```python
from build123d import *

# Parameters (mm, degrees)
F0_R     = 5.5626
F1_DEPTH = 20.6502
F2_R     = 19.05
F3_DEPTH = 31.75
F5_DEPTH = 68.2762


with BuildPart() as f1:
    # F0 (on Top) → F1 (new body)
    with BuildSketch(Plane.XY):
        with BuildLine():
            ThreePointArc((19.05, 30.048523), (6.35, 30.048523), (0, 19.05))
            Line((0, 19.05), (0, -19.05))
            ThreePointArc((0, -19.05), (6.35, -30.048523), (19.05, -30.048523))
            Line((19.05, -30.048523), (52.045568, -10.998523))
            ThreePointArc((52.045568, -10.998523), (58.395568, 0), (52.045568, 10.998523))
            Line((52.045568, 10.998523), (19.05, 30.048523))
        make_face()
        with Locations((12.7, -19.05)):
            Circle(F0_R, mode=Mode.SUBTRACT)
        with Locations((12.7, 19.05)):
            Circle(F0_R, mode=Mode.SUBTRACT)
        with Locations((45.695568, 0)):
            Circle(F0_R, mode=Mode.SUBTRACT)
    extrude(amount=F1_DEPTH)

    # F2 (on Front) → F3 (join, symmetric)
    with BuildSketch(Plane.XZ):
        with BuildLine():
            Line((12.7, 15.875), (-40.783613, 15.875))
            ThreePointArc((-40.783613, 15.875), (-61.435199, -39.990856), (-9.411603, -10.990385))
            ThreePointArc((-9.411603, -10.990385), (-7.234757, -3.329524), (0, 0))
            Line((0, 0), (12.7, 0))
            Line((12.7, 0), (12.7, 15.875))
        make_face()
        with Locations((-40.783613, -15.875)):
            Circle(F2_R, mode=Mode.SUBTRACT)
    extrude(amount=F3_DEPTH, both=True)

    # F4 (on face) → F5 (cut, through all)
    with BuildSketch(Plane.XY.offset(20.6502)):
        with BuildLine():
            Line((12.7, 13.4874), (12.7, 24.6126))
            ThreePointArc((12.7, 24.6126), (7.1374, 19.05), (12.7, 13.4874))
        make_face()
        with BuildLine():
            ThreePointArc((12.7, -13.4874), (7.1374, -19.05), (12.7, -24.6126))
            Line((12.7, -24.6126), (12.7, -13.4874))
        make_face()
    extrude(amount=-F5_DEPTH, mode=Mode.SUBTRACT)


solid = f1.part
```
Model file for the job. Use its own axes, mm. A direction names the side the tool comes from. Coordinates: 2 decimals unless noted, no trailing zeros. Order: outer loops, then holes, each group sorted by start corner. A loop starts at its lowest first (then second) coordinate and runs counter-clockwise, first axis right, second up. Notation, with made-up numbers: (69, -39) -> (82, -39) arc R16 cw to (82, -27) -> close; hole circle Ø4 at (23.25, 12). An arc over 180 degrees is marked (long way). Return JSON: item names as keys, results as strings.
Item 1: Slice it at C-C (z = -21.5). Write the cut outline in (x, y), then the cut area to 3 significant figures.
Model answer:
{"outline": "(-72.03, -31.75) -> (-58.98, -31.75) -> (-58.98, 31.75) -> (-72.03, 31.75) -> close; (-22.58, -31.75) -> (-9.54, -31.75) -> (-9.54, 31.75) -> (-22.58, 31.75) -> close", "area": "1,660 mm²"}
Item 2: Mould opens along Z. For faces 1 (the face through (-20, 0, 15.875)), 2 (the face through (51, 1.67, 10.18)), 3 (the face through (22, 0, 0)), 4 (the face through (-7.31, -0.44, -3.42)) say: pulls with the +Z half, pulls with the -Z half, needs draft (parallel to the pull), parting line crosses it, or undercut.
Model answer:
{"face 1": "pulls with the +Z half", "face 2": "needs draft", "face 3": "pulls with the -Z half", "face 4": "undercut"}
Item 3: Slice it at B-B (x = 42). Write the cut outline in (y, z).
Model answer:
{"outline": "(-16.8, 0) -> (-4.16, 0) -> (-4.16, 20.65) -> (-16.8, 20.65) -> close; (4.16, 0) -> (16.8, 0) -> (16.8, 20.65) -> (4.16, 20.65) -> close"}
Item 4: Slice it at A-A (y = 0). Write the cut outline in (x, z) (3 decimals), then the cut area to 3 significant figures.
Model answer:
{"outline": "(-40.784, 15.875) arc R31.75 ccw (long way) to (-9.412, -10.99) arc R9.525 cw to (0, 0) -> (40.133, 0) -> (40.133, 20.65) -> (0, 20.65) -> (0, 15.875) -> close; (51.258, 0) -> (58.396, 0) -> (58.396, 20.65) -> (51.258, 20.65) -> close; hole circle Ø38.1 at (-40.784, -15.875)", "area": "3,380 mm²"}
Item 5: 3-axis set-ups, long thin cutter, end or side, ignore diameter. For faces 5 (the face through (11.776, -31.716, 17.064)), 6 (the face through (-62.245, -0.444, -39.273)), 7 (the face through (12.15, 31.74, 17.06)), 8 (the face through (0, 0, 18)), 9 (the face through (18.006, -17.379, 10.181)): which of +Z, -Z, +X, -X, +Y, -Y reach the whole face in a straight line?
Model answer:
{"face 5": "+Z, -Y", "face 6": "+Y, -Y", "face 7": "+Z, +Y", "face 8": "+Z, -X, +Y, -Y", "face 9": "+Z, -Z"}
Item 6: Wall check: line 1 along Y through (x, z) = (12.7, 12); line 2 along Y through (x, z) = (12, 12); line 3 along Z through (x, y) = (8.5, 11.5). Give the ranges that are in metal, low to high. Write a range as from..to.
Model answer:
{"line 1": "y = -31.75..-24.61, -13.49..13.49, 24.61..31.75", "line 2": "y = -31.75..-24.57, -13.53..13.53, 24.57..31.75", "line 3": "z = 0..20.65"}
Item 7: Pin check, flat tips, straight feed: P1, Ø14.5, axis at x = 12.7, y = 19.05, coming from the -Z side; P2, Ø5, axis at y = -1, z = -6.5, coming from the +X side; P3, Ø2, axis at y = -20, z = -23, coming from the -X side; P4, Ø23, axis at x = -40.78, z = -15.88, coming from the -Y side. Stop position of each tip, or through.
Model answer:
{"P1": "stops at z = 0", "P2": "stops at x = -7.76", "P3": "stops at x = -71.94", "P4": "passes through"}
Item 8: Slice it at D-D (y = 22.5). Write the cut outline in (x, z) (3 decimals), then the cut area to 3 significant figures.
Model answer:
{"outline": "(-40.784, 15.875) arc R31.75 ccw (long way) to (-9.412, -10.99) arc R9.525 cw to (0, 0) -> (8.337, 0) -> (8.337, 20.65) -> (0.478, 20.65) -> (0.478, 15.875) -> close; (17.063, 0) -> (32.124, 0) -> (32.124, 20.65) -> (17.063, 20.65) -> close; hole circle Ø38.1 at (-40.784, -15.875)", "area": "2,880 mm²"}
